Study the drawing (mm; zero at the part's minimum x, y, z) and answer. A direction names the side the tool comes from. Give positions to 0.01 mm unless a question says otherwise; leave off trailing zeros. Order: outer loops, then holes, each group sorted by start corner. A loop starts at its lowest first (then second) coordinate and runs counter-clockwise, first axis right, second up. Notation, with made-up numbers: (50.5, 32.5) -> (94.5, 32.5) arc R36 ccw to (94.5, 68.5) -> close; hole circle Ø4 at (70.5, 48). An arc over 180 degrees is marked (long way). Answer as CSV lines item,"result". Start each with the question number.
1. For the marked faces 1, 2, 3 and 4, determine the directions among +Z, -Z, +X, -X, +Y, -Y from which every point of the face is accessible in a straight line to the end or side of a thin tool.
2. Find the intervals of material crossed by L1, parallel to X at y = 1, z = 125; L2, parallel to Z at x = 95, y = 2.15; L3, parallel to X at y = 10.5, z = 124.5, in increasing order.
3. Flat-ended cylindrical pins translate along their axes: pin 1 (22 mm diameter, centred on x = 46, y = 30, fed in from -Z); pin 2 (20 mm diameter, centred on y = 20, z = 111.5, fed in from -X); pin 3 (4 mm diameter, centred on x = 99, y = 8, fed in from -Z). Find the tip coordinate at first contact, or state that the pin passes through.
4. A cutting plane is placed at D-D (z = 125). Give the vertices of the cut face in (x, y).
5. A cutting plane is placed at A-A (z = 5). Give the vertices of the cut face in (x, y).
6. A cutting plane is placed at B-B (y = 17). Give the vertices of the cut face in (x, z).
7. A cutting plane is placed at C-C (x = 75). Give the vertices of the cut face in (y, z), then the cut area to 3 significant figures.
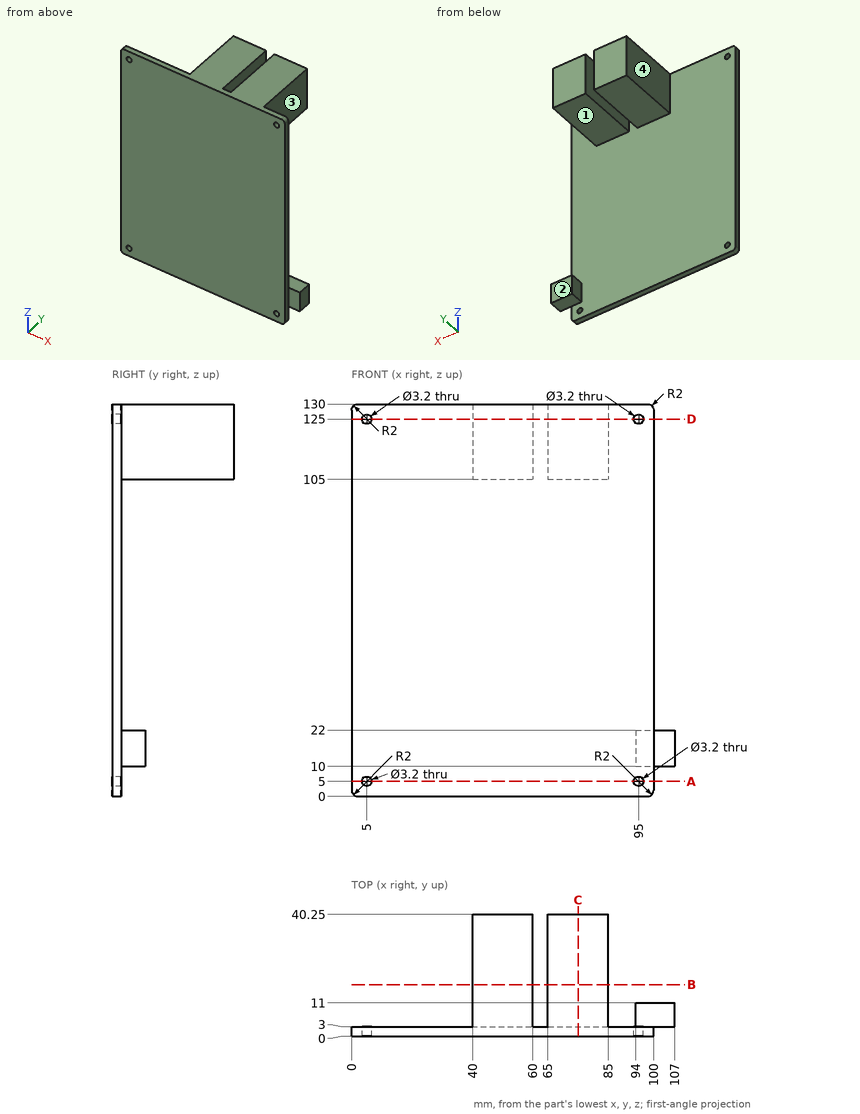
Answer sheet:
1,face 1,"-Z, +X, -X, +Y"
1,face 2,"+Z, -Z, +X, -X, +Y"
1,face 3,"+Z, -Z, +X, +Y"
1,face 4,"+Z, -Z, -X, +Y"
2,L1,"x = 0 to 3.4, 6.6 to 93.4, 96.6 to 100"
2,L2,"z = 0 to 3.4, 6.6 to 123.4, 126.6 to 130"
2,L3,"x = 40 to 60, 65 to 85"
3,pin 1,"stops at z = 105"
3,pin 2,"stops at x = 40"
3,pin 3,"stops at z = 10"
4,outline,"(0, 0) -> (3.4, 0) -> (3.4, 3) -> (0, 3) -> close; (6.6, 0) -> (93.4, 0) -> (93.4, 3) -> (85, 3) -> (85, 40.25) -> (65, 40.25) -> (65, 3) -> (60, 3) -> (60, 40.25) -> (40, 40.25) -> (40, 3) -> (6.6, 3) -> close; (96.6, 0) -> (100, 0) -> (100, 3) -> (96.6, 3) -> close"
5,outline,"(0, 0) -> (3.4, 0) -> (3.4, 3) -> (0, 3) -> close; (6.6, 0) -> (93.4, 0) -> (93.4, 3) -> (6.6, 3) -> close; (96.6, 0) -> (100, 0) -> (100, 3) -> (96.6, 3) -> close"
6,outline,"(40, 105) -> (60, 105) -> (60, 130) -> (40, 130) -> close; (65, 105) -> (85, 105) -> (85, 130) -> (65, 130) -> close"
7,outline,"(0, 0) -> (3, 0) -> (3, 105) -> (40.25, 105) -> (40.25, 130) -> (0, 130) -> close"
7,area,"1,320 mm^2"
